Design review of the part built by this model. Coordinates are the model's own, in mm. A direction names the side the tool comes from. Coordinates: 2 decimals unless noted, no trailing zeros. Answer in a Markdown table with one row per item.
Autodesk Inventor part; units mm, degrees
ref_plane "YZ Plane" through (0, 0, 0) normal (1, 0, 0) x (0, 1, 0)
ref_plane "XZ Plane" through (0, 0, 0) normal (0, 1, 0) x (-1, 0, 0)
ref_plane "XY Plane" through (0, 0, 0) normal (0, 0, 1) x (1, 0, 0)
sketch "Sketch1" plane through (0, 0, 0) normal (0, 1, 0) x (-1, 0, 0)
  line L0 (312.1225, 324.0216) -> (-94.2775, 324.0216)
  line L1 (-94.2775, 324.0216) -> (-94.2775, -158.5784)
  line L2 (-94.2775, -158.5784) -> (312.1225, -158.5784)
  line L3 (312.1225, -158.5784) -> (312.1225, 324.0216)
  point P0 (0, 0)
  dimension "d0" = 406.4
  dimension "d1" = 482.6
extrude "Board" add sketch "Sketch1" along normal blind 25.4
sketch "Hinge Cuts" plane through (0, 25.4, 0) normal (0, 1, 0) x (1, 0, 0)
  line L0 (-312.1225, 158.5784) -> (-312.1225, -324.0216)
  line L1 (-312.1225, 56.9784) -> (-300.9973, 56.9784)
  line L2 (-297.8223, 53.8034) -> (-297.8223, 22.0534)
  line L3 (-300.9973, 18.8784) -> (-312.1225, 18.8784)
  line L4 (-312.1225, 18.8784) -> (-312.1225, 56.9784)
  line L5 (94.2775, 158.5784) -> (-312.1225, 158.5784)
  line L6 (-312.1225, -222.4216) -> (-300.9973, -222.4216)
  line L7 (-297.8223, -219.2466) -> (-297.8223, -187.4966)
  line L8 (-300.9973, -184.3216) -> (-312.1225, -184.3216)
  line L9 (-312.1225, -184.3216) -> (-312.1225, -222.4216)
  arc A0 (-297.8223, -187.4966) -> (-300.9973, -184.3216) centre (-300.9973, -187.4966) ccw
  arc A1 (-300.9973, -222.4216) -> (-297.8223, -219.2466) centre (-300.9973, -219.2466) ccw
  arc A2 (-300.9973, 18.8784) -> (-297.8223, 22.0534) centre (-300.9973, 22.0534) ccw
  arc A3 (-297.8223, 53.8034) -> (-300.9973, 56.9784) centre (-300.9973, 53.8034) ccw
  point P0 (0, 0)
  point P1 (-297.8223, 18.8784)
  point P2 (-297.8223, 56.9784)
  point P3 (-297.8223, -184.3216)
  point P4 (-297.8223, -222.4216)
  dimension "d4" = 38.1
  dimension "d5" = 14.3002
  dimension "d6" = 101.6
  dimension "d7" = 38.1
  dimension "d8" = 14.3002
  dimension "d9" = 203.2
  dimension "d10" = 3.175
extrude "Extrusion2" cut sketch "Hinge Cuts" against normal blind 3.175
equation "\"d6\" = 0.25 * d1 - 0.5 * d4"
equation "\"d9\" = 2 * d6"
properties part number "Extension Shelves" material "Wood (Oak)"
(1) Insertion check: pin 1 Ø1 at (y, z) = (24, 200) entering from -X; pin 2 Ø4.5 at (x, z) = (-308, -42) entering from +Y (3 decimals). Each pin has a flat end and moves straight along its axis. Give the tip position at first contact, or say it passes through.
Return value:
| item | result |
|---|---|
| pin 1 | stops at x = -297.82 |
| pin 2 | stops at y = 22.225 |
(2) For faces 5 (the flat face through (-106, 25.4, 86)), 6 (the flat face through (-305, 22.225, 203)), list the 3-axis set-ups (+Z, -Z, +X, -X, +Y, -Y) from which the entire face can be reached by the end or side of a thin tool; tool diameter is ignored.
Return value:
| item | result |
|---|---|
| face 5 | +Z, -Z, +X, -X, +Y |
| face 6 | -X, +Y |
(3) Draft analysis for pull direction Z (two halves, no side actions). For faces 1 (the flat face through (-112, 13, 324.022)), 2 (the flat face through (-305, 22.225, -38)), 3 (the flat face through (-312.122, 13, 79)), 4 (the flat face through (-106, 13, -158.578)), state which applies: pulls with the +Z half, pulls with the -Z half, needs draft (parallel to the pull), parting line crosses it, or undercut.
Return value:
| item | result |
|---|---|
| face 1 | pulls with the +Z half |
| face 2 | undercut |
| face 3 | needs draft |
| face 4 | pulls with the -Z half |
